The model under review builds one solid part; all positions refer to its coordinate system, in mm. Face numbers are marked on the shaded views. A direction names the side the tool comes from. Round coordinates to 2 decimals unless told otherwise and drop trailing zeros. Write each loop counter-clockwise with the first axis right and the second up, starting at its lowest first coordinate (ties: lowest second). Pieces come first, ordered by that corner, then holes. Notation, with made-up numbers: (-5.75, 64) - (51.25, 64) arc R8 cw to (51.25, 79) - close; hole circle Ø8 at (61.25, -15.75). An arc over 180 degrees is marked (long way). Use one line per item in the form item = value.
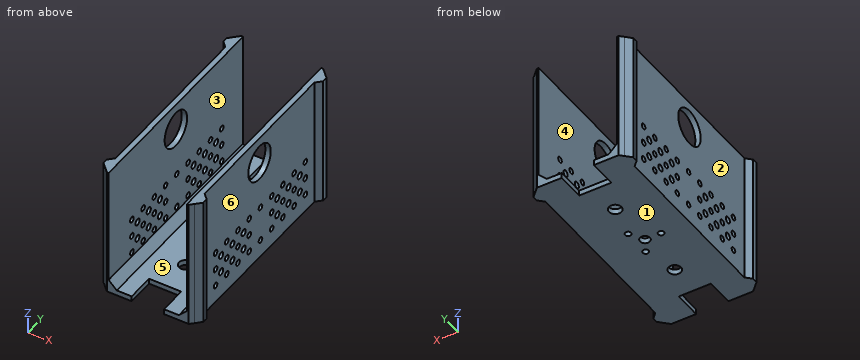
from build123d import *

# Parameters (mm, degrees)
BOSS_EXTRUDE1_DEPTH = 3
BOSS_EXTRUDE2_DEPTH = 70
SKETCH3_R           = 1.65
SKETCH3_R_2         = 2.75
SKETCH3_R_3         = 3.5
CUT_EXTRUDE1_DEPTH  = 3
CHAMFER1_SIZE       = 4.5
CHAMFER2_SIZE       = 3
SKETCH4_R           = 10
SKETCH4_R_2         = 1.6
SKETCH4_R_3         = 1.842058484
CUT_EXTRUDE2_DEPTH  = 138.709585723
CHAMFER3_SIZE       = 2


with BuildPart() as part:
    # Sketch1 → Boss-Extrude1 (new body)
    with BuildSketch(Plane.XY):
        Polygon((9, 0), (-9, 0), (-9, -15.5), (-24.85, -15.5), (-24.85, -10.5), (-27.85, -10.5), (-27.85, -7.5), (-24.85, -7.5), (-24.85, 36.35), (-24.85, 41.85), (-24.85, 46.85), (-24.85, 52.35), (-24.85, 96.2), (-27.85, 96.2), (-27.85, 99.2), (-24.85, 99.2), (-24.85, 104.2), (-9, 104.2), (-9, 88.7), (9, 88.7), (9, 104.2), (24.85, 104.2), (24.85, 99.2), (27.85, 99.2), (27.85, 96.2), (24.85, 96.2), (24.85, 52.35), (24.85, 46.85), (24.85, 41.85), (24.85, 36.35), (24.85, -7.5), (27.85, -7.5), (27.85, -10.5), (24.85, -10.5), (24.85, -15.5), (9, -15.5), align=None)
    extrude(amount=BOSS_EXTRUDE1_DEPTH)

    # Sketch2 → Boss-Extrude2 (add)
    with BuildSketch(Plane.XY.offset(3)):
        Polygon((-24.85, 104.2), (-21.85, 104.2), (-21.85, -15.5), (-24.85, -15.5), (-24.85, -10.5), (-27.85, -10.5), (-27.85, -7.5), (-24.85, -7.5), (-24.85, 96.2), (-27.85, 96.2), (-27.85, 99.2), (-24.85, 99.2), align=None)
        Polygon((21.85, 104.2), (21.85, -15.5), (24.85, -15.5), (24.85, -10.5), (27.85, -10.5), (27.85, -7.5), (24.85, -7.5), (24.85, 96.2), (27.85, 96.2), (27.85, 99.2), (24.85, 99.2), (24.85, 104.2), align=None)
    extrude(amount=BOSS_EXTRUDE2_DEPTH)

    # Sketch3 → Cut-Extrude1 (cut)
    with BuildSketch(Plane(origin=(0, 0, 0), x_dir=(-1, 0, 0), z_dir=(0, 0, -1))):
        with Locations((9, 44.35)):
            Circle(SKETCH3_R)
        with Locations((-4.5, 36.555771366)):
            Circle(SKETCH3_R)
        with Locations((-4.5, 52.144228634)):
            Circle(SKETCH3_R)
        with Locations((0, 44.35)):
            Circle(SKETCH3_R_2)
        with Locations((0, 70.85)):
            Circle(SKETCH3_R_3)
        with Locations((0, 17.85)):
            Circle(SKETCH3_R_3)
    extrude(amount=-CUT_EXTRUDE1_DEPTH, mode=Mode.SUBTRACT)

    # Chamfer1
    chamfer1_edges = [part.edges().sort_by_distance(p)[0] for p in [
        (-21.85, 44.35, 3),
        (21.85, 44.35, 3),
    ]]
    chamfer(chamfer1_edges, length=CHAMFER1_SIZE)

    # Chamfer2
    chamfer2_edges = [part.edges().sort_by_distance(p)[0] for p in [
        (24.85, 99.2, 36.5),
        (24.85, 96.2, 36.5),
        (24.85, -10.5, 36.5),
        (24.85, -7.5, 36.5),
        (-24.85, -7.5, 36.5),
        (-24.85, -10.5, 36.5),
        (-24.85, 99.2, 36.5),
        (-24.85, 96.2, 36.5),
    ]]
    chamfer(chamfer2_edges, length=CHAMFER2_SIZE - 0.0001)  # a hair under: the kernel refuses the full size

    # Sketch4 → Cut-Extrude2 (cut, through all)
    with BuildSketch(Plane.ZY.offset(24.85)):
        with Locations((58, 44.35)):
            Circle(SKETCH4_R)
        with Locations((10, 85.2)):
            Circle(SKETCH4_R_2)
        with Locations((20, 85.2)):
            Circle(SKETCH4_R_2)
        with Locations((30, 85.2)):
            Circle(SKETCH4_R_2)
        with Locations((20, 75.2)):
            Circle(SKETCH4_R_2)
        with Locations((30, 75.2)):
            Circle(SKETCH4_R_2)
        with Locations((20, 65.2)):
            Circle(SKETCH4_R_2)
        with Locations((30, 65.2)):
            Circle(SKETCH4_R_2)
        with Locations((20, 55.2)):
            Circle(SKETCH4_R_2)
        with Locations((30, 55.2)):
            Circle(SKETCH4_R_2)
        with Locations((30, 45.2)):
            Circle(SKETCH4_R_2)
        with Locations((20, 35.2)):
            Circle(SKETCH4_R_2)
        with Locations((30, 35.2)):
            Circle(SKETCH4_R_2)
        with Locations((20, 25.2)):
            Circle(SKETCH4_R_2)
        with Locations((30, 25.2)):
            Circle(SKETCH4_R_2)
        with Locations((20, 15.2)):
            Circle(SKETCH4_R_2)
        with Locations((30, 15.2)):
            Circle(SKETCH4_R_2)
        with Locations((20, 5.2)):
            Circle(SKETCH4_R_2)
        with Locations((30, 5.2)):
            Circle(SKETCH4_R_2)
        with Locations((10, 75.2)):
            Circle(SKETCH4_R_2)
        with Locations((10, 65.2)):
            Circle(SKETCH4_R_2)
        with Locations((10, 55.2)):
            Circle(SKETCH4_R_2)
        with Locations((10, 45.2)):
            Circle(SKETCH4_R_2)
        with Locations((10, 35.2)):
            Circle(SKETCH4_R_2)
        with Locations((10, 25.2)):
            Circle(SKETCH4_R_2)
        with Locations((10, 15.2)):
            Circle(SKETCH4_R_2)
        with Locations((10, 5.2)):
            Circle(SKETCH4_R_2)
        with Locations((15, 80.2)):
            Circle(SKETCH4_R_3)
        with Locations((25, 80.2)):
            Circle(SKETCH4_R_3)
        with Locations((25, 70.2)):
            Circle(SKETCH4_R_3)
        with Locations((25, 60.2)):
            Circle(SKETCH4_R_3)
        with Locations((25, 30.2)):
            Circle(SKETCH4_R_3)
        with Locations((25, 20.2)):
            Circle(SKETCH4_R_3)
        with Locations((25, 10.2)):
            Circle(SKETCH4_R_3)
        with Locations((15, 70.2)):
            Circle(SKETCH4_R_3)
        with Locations((15, 60.2)):
            Circle(SKETCH4_R_3)
        with Locations((15, 30.2)):
            Circle(SKETCH4_R_3)
        with Locations((15, 20.2)):
            Circle(SKETCH4_R_3)
        with Locations((15, 10.2)):
            Circle(SKETCH4_R_3)
    extrude(amount=-CUT_EXTRUDE2_DEPTH, mode=Mode.SUBTRACT)

    # Chamfer3
    chamfer3_edges = [part.edges().sort_by_distance(p)[0] for p in [
        (24.85, -15.5, 36.5),
        (-24.85, -15.5, 36.5),
        (24.85, 104.2, 36.5),
        (-24.85, 104.2, 36.5),
    ]]
    chamfer(chamfer3_edges, length=CHAMFER3_SIZE)


solid = part.part
(1) Machinability: for the marked faces 5 and 6, which of the approach directions +Z, -Z, +X, -X, +Y, -Y give a long, thin tool a straight path to every point of the face, cutting with its end or side? Answer none if there is none.
Geometry results:
face_5 = +Z, +Y, -Y
face_6 = +Z, -Z, +X
(2) The part is to be moulded in two halves that separate along X. For the marked faces 1, 2, 3 and 4, say which applies: +X half, -X half, draft (parallel to the pull), parting line (faces both ways), or undercut.
Geometry results:
face_1 = draft
face_2 = -X half
face_3 = undercut
face_4 = undercut
(3) Add section A-A on y = 91. Write out the cut boundary in (x, z).
Geometry results:
outline = (-24.85, 0) - (-9, 0) - (-9, 3) - (-17.35, 3) - (-21.85, 7.5) - (-21.85, 73) - (-24.85, 73) - close; (9, 0) - (24.85, 0) - (24.85, 73) - (21.85, 73) - (21.85, 7.5) - (17.35, 3) - (9, 3) - close
(4) Insertion check: P1, Ø5, axis at y = 35.2, z = 20, coming from the +X side; P2, Ø1.5, axis at x = 19.5, z = 52.5, coming from the -Y side; P3, Ø4, axis at y = 10.2, z = 25, coming from the -X side; P4, Ø2, axis at x = 10, y = 17.5, coming from the +Z side. Each pin has a flat end and moves straight along its axis. Give the tip position at first contact, or say it passes through.
Geometry results:
P1 = 24.85
P2 = through
P3 = -24.85
P4 = 3
(5) Add section C-C on z = 20. Count the separate pieces of the cut face and the enclosed holes in it, then the cut area to 3 significant figures.
Geometry results:
separate_pieces = 18
enclosed_holes = 0
area = 629 mm2
(6) Add section B-B on x = 0. Write out the cut boundary in (y, z), then the cut area to 3 significant figures.
Geometry results:
outline = (0, 0) - (14.35, 0) - (14.35, 3) - (0, 3) - close; (21.35, 0) - (41.6, 0) - (41.6, 3) - (21.35, 3) - close; (47.1, 0) - (67.35, 0) - (67.35, 3) - (47.1, 3) - close; (74.35, 0) - (88.7, 0) - (88.7, 3) - (74.35, 3) - close
area = 208 mm2
(7) To check wall thickness, follow L1, parallel to Z at x = 23, y = 75; L2, parallel to Z at x = -22, y = 60; L3, parallel to X at y = 45, z = 13. State the ranges of each line that lie inside material, in increasing order.
Geometry results:
L1 = 0 to 8.41, 11.59 to 18.41, 21.59 to 28.41, 31.59 to 73
L2 = 0 to 13.17, 16.83 to 23.17, 26.83 to 73
L3 = -24.85 to -21.85, 21.85 to 24.85
